Design review of the part built by this model. Coordinates are the model's own, in mm. Face numbers are marked on the shaded views. A direction names the side the tool comes from. Coordinates: 2 decimals unless noted, no trailing zeros. Order: outer loops, then holes, each group sorted by start corner. A loop starts at its lowest first (then second) coordinate and runs counter-clockwise, first axis right, second up. Notation, with made-up numbers: (-7.5, 76.5) -> (4.5, 76.5) arc R22 ccw to (4.5, 115.5) -> close; hole circle Ø1 at (2, -8.75). An arc over 180 degrees is marked (long way). Write item = value, one per line.
Autodesk Inventor part; units mm, degrees
sketch "Boceto1" plane through (0, 0, 0) normal (0, 0, 1) x (1, 0, 0)
  line L0 (-12, 0) -> (12, 0)
  line L1 (15, -3) -> (15, -22.1495)
  line L2 (-15, -22.1495) -> (-15, -3)
  line L3 (12, 0) -> (15, -3)
  line L4 (-12, 0) -> (-15, -3)
  line L5 (-15, -22.1495) -> (-4.9497, -32.1997)
  arc A0 (-4.9497, -32.1997) -> (4.9497, -32.1997) centre (0, -27.25) ccw
  line L6 (4.9497, -32.1997) -> (15, -22.1495)
  point P0 (0, 0)
  point P1 (-15, 0)
  point P2 (15, 0)
  point P3 (0, 0)
  point P4 (0, -34.25)
  point P5 (15, 0)
  point P6 (0, -34.25)
  dimension "d0" = 30
  dimension "d5" = 3
  dimension "d6" = 3
  dimension "d10" = 135
  dimension "d55" = 27.25
  dimension "d59" = 7
  dimension "d60" = 34.25
extrude "Extrusión1" add sketch "Boceto1" along normal blind 10
sketch "Boceto2" plane through (0, 0, 10) normal (0, 0, 1) x (1, 0, 0)
  line L0 (15, -22.1495) -> (15, -3)
  line L1 (15, -3) -> (12, 0)
  line L2 (12, 0) -> (-12, 0)
  line L3 (-12, 0) -> (-15, -3)
  line L4 (-15, -3) -> (-15, -22.1495)
  line L5 (-15, -22.1495) -> (-4.9497, -32.1997)
  arc A0 (-4.9497, -32.1997) -> (4.9497, -32.1997) centre (0, -27.25) ccw
  line L6 (4.9497, -32.1997) -> (15, -22.1495)
  line L7 (-15, -19.5) -> (-12, -22.5)
  line L8 (-12, -22.5) -> (12, -22.5)
  line L9 (12, -22.5) -> (15, -19.5)
  point P0 (0, 0)
  dimension "d13" = 3
  dimension "d14" = 3
  dimension "d15" = 3
  dimension "d16" = 3
  dimension "d17" = 22.5
extrude "Extrusión2" add sketch "Boceto2" along normal blind 9.25 contours L9 L8 L7 L4 L3 L2 L1 L0
sketch "Boceto3" plane through (15, -22.1495, 0) normal (1, 0, 0) x (0, 0, -1)
  line L0 (-19.25, 2.6495) -> (-19.25, 19.1495)
  line L1 (-19.25, 19.1495) -> (-19.25, 2.6495)
  line L2 (-19.25, 3.6495) -> (-14.25, 3.6495)
  arc A0 (-14.25, 3.6495) -> (-14.25, 18.1495) centre (-14.25, 10.8995) ccw
  line L3 (-14.25, 18.1495) -> (-19.25, 18.1495)
  point P0 (0, 22.1495)
  point P1 (-7, 10.8995)
  point P2 (-19.25, 10.8995)
  dimension "d20" = 12.25
  dimension "d21" = 14.5
extrude "Extrusión3" cut sketch "Boceto3" against normal through all
hole "Agujero1" at (0, -27.25, 0) direction (0, 0, 1) diameter 3.75 depth 8 tip angle 118
ref_plane "Plano de trabajo1" through (0, 0, 4) normal (0, 0, 1) x (1, 0, 0)
sketch "Boceto4" plane through (0, 0, 4) normal (0, 0, 1) x (1, 0, 0)
  circle A0 centre (0, -27.25) radius 1.875
  line L0 (0, -23.6502) -> (3.1175, -25.4501)
  line L1 (3.1175, -25.4501) -> (3.1175, -29.0499)
  line L2 (-3.1175, -29.0499) -> (-3.1175, -25.4501)
  line L3 (-3.1175, -25.4501) -> (0, -23.6502)
  line L4 (-3.1175, -29.0499) -> (-3.1175, -35.0499)
  line L5 (-3.1175, -35.0499) -> (3.1175, -35.0499)
  line L6 (3.1175, -35.0499) -> (3.1175, -29.0499)
  point P0 (0, 0)
  point P1 (0, -27.25)
  dimension "d36" = 6.235
  dimension "d37" = 6
extrude "Extrusión4" cut sketch "Boceto4" along normal blind 3
sketch "Boceto5" plane through (0, 0, 0) normal (1, 0, 0) x (0, 1, 0)
  arc A0 (-18.5, 14.25) -> (-4, 14.25) centre (-11.25, 14.25) ccw
  circle A1 centre (-11.25, 16.25) radius 11.5
  circle A2 centre (-11.25, 16.25) radius 13.5
  point P0 (0, 0)
  dimension "d44" = 27
  dimension "d45" = 23
  dimension "d46" = 2
extrude "Extrusión5" cut sketch "Boceto5" along normal mid plane 4.5
sketch "Boceto6" plane through (0, 0, 0) normal (1, 0, 0) x (0, 1, 0)
  line L0 (-18.5, 19.25) -> (-19.5, 19.25)
  arc A0 (-18.5, 14.25) -> (-4, 14.25) centre (-11.25, 14.25) ccw
  circle A1 centre (-11.25, 14.25) radius 7.6
  point P0 (0, 0)
  dimension "d49" = 15.2
extrude "Extrusión6" cut sketch "Boceto6" along normal mid plane 24.2
ref_plane "Plano de trabajo2" through (15, -11.25, 14.25) normal (0, -1, 0) x (1, 0, 0)
sketch "Boceto7" plane through (15, -11.25, 14.25) normal (0, -1, 0) x (1, 0, 0)
  line L0 (-10.0503, -14.25) -> (0, -14.25)
  line L1 (0, -14.25) -> (0, -4.25)
  line L2 (-10.0503, -4.25) -> (0, -4.25)
  line L3 (-10.0503, -14.25) -> (-10.0503, -4.25)
  line L4 (-2.9, -7.6) -> (-2.9, 2.2798)
  line L5 (-2.9, 0) -> (-2.9, 0)
  line L6 (0, 0) -> (-2.9, 0)
  line L7 (0, 0) -> (0, 0)
  line L8 (0, 0) -> (-2.9, 0)
  line L9 (-2.9, -7.3639) -> (-1.67, -7.2479)
  line L10 (-1.67, -7.2479) -> (-2.9, -7.2479)
  line L11 (-2.9, -7.3639) -> (-2.9, -7.2479)
  point P0 (-15, -14.25)
  dimension "d52" = 0.116
  dimension "d53" = 1.23
revolve "Revolución1" cut sketch "Boceto7" angle 360 about axis through (15, -11.25, 14.25) along (-1, 0, 0) contours L10 L9 L4
mirror "Simetría1" about plane through (0, 0, 0) normal (1, 0, 0) of "Revolución1"
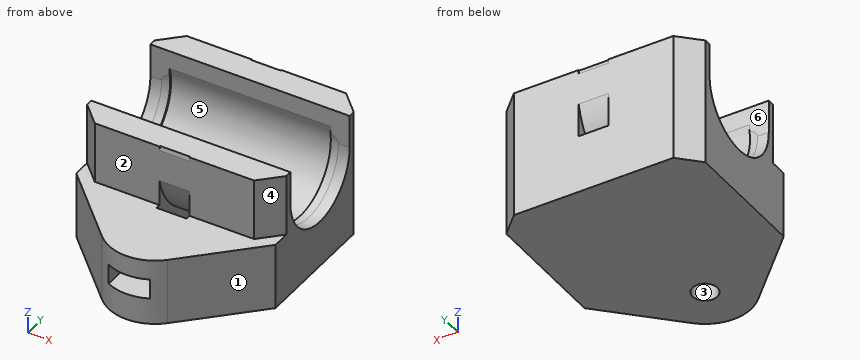
(1) We need section A-A (z = 17). Write out the cut boundary in (x, y).
Report:
outline = (-15, -19.5) -> (-12, -22.5) -> (12, -22.5) -> (15, -19.5) -> (15, -18.5) -> (-15, -18.5) -> close; (-15, -4) -> (15, -4) -> (15, -3) -> (12, 0) -> (-12, 0) -> (-15, -3) -> close
(2) For the marked faces 4, 5 and 6, list the 3-axis set-ups (+Z, -Z, +X, -X, +Y, -Y) from which the entire face can be reached by the end or side of a thin tool; tool diameter is ignored.
Report:
face_4 = +Z, +X, -Y
face_5 = none
face_6 = +Z, +X, -X
(3) For L1, parallel to X at y = -7, z = 5; L2, parallel to Z at x = 3.5, y = -23; L3, parallel to Y at x = -1.5, z = 9.75, list the stretches that pass through material, from the lowest coordinate up.
Report:
L1 = -15 to -2.25, 2.25 to 15
L2 = 0 to 10
L3 = -34.09 to -23.08, -20.74 to -17.37, -5.13 to -1.76
(4) Insertion check: pin 1 (2.5 mm diameter, centred on x = 4, z = 16, fed in from -Y); pin 2 (1 mm diameter, centred on x = 0.5, z = 11.5, fed in from -Y); pin 3 (2.5 mm diameter, centred on y = -30.5, z = 6, fed in from -X). Each pin has a flat end and moves straight along its axis. Give the tip position at first contact, or say it passes through.
Report:
pin_1 = -22.5
pin_2 = -21.94
pin_3 = -7.9
(5) We need section B-B (y = -11.25). Write out the cut boundary in (x, z), and give its area (3 significant figures).
Report:
outline = (-15, 0) -> (15, 0) -> (15, 7) -> (13.31, 7) -> (12.1, 6.89) -> (12.1, 6.65) -> (-12.1, 6.65) -> (-12.1, 6.89) -> (-13.31, 7) -> (-15, 7) -> close; hole (-2.25, 2.75) -> (2.25, 2.75) -> (2.25, 4.75) -> (-2.25, 4.75) -> close
area = 192 mm²
(6) The part is to be moulded in two halves that separate along X. For the marked faces 1, 2 and 3, say which applies: released by +X, released by -X, zero draft, split by the parting line, or undercut.
Report:
face_1 = released by +X
face_2 = zero draft
face_3 = undercut
